```python
from build123d import *

# Parameters (mm, degrees)
SKETCH001_W  = 31.8
SKETCH001_H  = 7.8
PAD_DEPTH    = 1.5
SKETCH002_R  = 2.5
PAD001_DEPTH = 2
FILLET_R     = 0.5
PAD002_DEPTH = 4.5
SKETCH004_W  = 5
SKETCH004_H  = 1.6
POCKET_DEPTH = 100


with BuildPart() as part:
    # Sketch001 → Pad (new body)
    with BuildSketch(Plane.XY):
        with Locations((16, 4)):
            Rectangle(SKETCH001_W, SKETCH001_H)
    extrude(amount=-PAD_DEPTH)

    # Sketch002 → Pad001 (join)
    with BuildSketch(Plane.XY):
        with Locations((4, 4)):
            Circle(SKETCH002_R)
        with Locations((12, 4)):
            Circle(SKETCH002_R)
        with Locations((20, 4)):
            Circle(SKETCH002_R)
        with Locations((28, 4)):
            Circle(SKETCH002_R)
    extrude(amount=PAD001_DEPTH)

    # Fillet
    fillet_edges = [part.edges().sort_by_distance(p)[0] for p in [
        (1.5, 4, 2),
        (9.5, 4, 2),
        (17.5, 4, 2),
        (25.5, 4, 2),
    ]]
    fillet(fillet_edges, radius=FILLET_R)

    # Sketch003 → Pad002 (join)
    with BuildSketch(Plane.XY):
        Polygon((0.1, 7.9), (31.9, 7.9), (31.9, 3), (29.9, 3), (29.9, 6.5), (17, 6.5), (17, 3), (15, 3), (15, 6.5), (2.1, 6.5), (2.1, 3), (0.1, 3), align=None)
        Polygon((0.1, 0.1), (0.1, 1.5), (7.05, 1.5), (7.05, 5), (9.05, 5), (9.05, 1.5), (22.95, 1.5), (22.95, 5), (24.95, 5), (24.95, 1.5), (31.9, 1.5), (31.9, 0.1), align=None)
    extrude(amount=-PAD002_DEPTH)

    # Sketch004 → Pocket (cut)
    with BuildSketch(Plane.YZ):
        with Locations((4, -2.3)):
            Rectangle(SKETCH004_W, SKETCH004_H)
    extrude(amount=POCKET_DEPTH, mode=Mode.SUBTRACT)


solid = part.part
```
Read the model definition and answer for the solid it produces. Units are mm, in the model's axes. A direction names the side the tool comes from. Give positions to 0.01 mm unless a question says otherwise; leave off trailing zeros. Loops run counter-clockwise (first coordinate to the right, second up) from the corner with the lowest first, then second, coordinate; pieces in that order, holes last.
Item 1: Find the intervals of material crossed by line 1 along X through (y, z) = (6, -3.5); line 2 along Y through (x, z) = (6, -3.25); line 3 along X through (y, z) = (3, 0.25), in increasing order.
Item 2: The mould has two halves that part along Z. Classify faces 4 (the flat face through (1, 3, -4)), 5 (the flat face through (16, 4, 0)), 6 (the flat face through (24, 3, -3.1)): released by +Z, released by -Z, zero draft, split by the parting line, or undercut.
Item 3: The part is cut by section D-D (x = 8). Write down the section's boundary in (y, z).
Item 4: The part is cut by section B-B (x = 28). Write down the section's boundary in (y, z), and give its area (3 significant figures).
Item 5: The part is cut by section A-A (z = -2.5). Write down the section's boundary in (x, y), and give its area (3 significant figures).
Item 6: This flat-tipped pin is pushed along its axis until it touches: pin 1 Ø1.6 at (x, y) = (8.5, 4) entering from +Z. Where does it stop, or does it pass through?
Item 7: For faces 1 (the flat face through (2.1, 5, -4)), 2 (the flat face through (15.8, 6.5, -2.7)), 3 (the cylindrical face through (26.16, 5.69, 0.74)), determine the directions among +Z, -Z, +X, -X, +Y, -Y from which every point of the face is accessible in a straight line to the end or side of a thin tool.
Item 8: The part is cut by section C-C (y = 4). Give the number of separate pieces and of enclosed holes in the cut face, and give its area (3 significant figures).
Taken from the geometry:
1. line 1: x = 0.1 to 2.1, 15 to 17, 29.9 to 31.9
1. line 2: y = 0.1 to 1.5, 6.5 to 7.9
1. line 3: x = 1.71 to 6.29, 9.71 to 14.29, 17.71 to 22.29, 25.71 to 30.29
2. face 4: zero draft
2. face 5: released by +Z
2. face 6: undercut
3. outline: (0.1, -4.5) - (5, -4.5) - (5, -3.1) - (1.5, -3.1) - (1.5, -1.5) - (6.5, -1.5) - (6.5, -4.5) - (7.9, -4.5) - (7.9, 0) - (0.1, 0) - close
4. outline: (0.1, -4.5) - (1.5, -4.5) - (1.5, -1.5) - (6.5, -1.5) - (6.5, -4.5) - (7.9, -4.5) - (7.9, 0) - (6.5, 0) - (6.5, 1.5) arc R0.5 ccw to (6, 2) - (2, 2) arc R0.5 ccw to (1.5, 1.5) - (1.5, 0) - (0.1, 0) - close
4. area: 30.0 mm2
5. outline: (0.1, 0.1) - (31.9, 0.1) - (31.9, 1.5) - (0.1, 1.5) - close; (0.1, 6.5) - (31.9, 6.5) - (31.9, 7.9) - (0.1, 7.9) - close
5. area: 89.0 mm2
6. pin 1: stops at z = 0
7. face 1: -Z
7. face 2: none
7. face 3: +Z
8. separate pieces: 6
8. enclosed holes: 0
8. area: 101 mm2
